Check sheet for the drawn part. Datum: minimum x, y, z corner. Units: mm. A direction names the side the tool comes from. Coordinates: 2 decimals unless noted, no trailing zeros. Order: outer loops, then holes, each group sorted by start corner. A loop starts at its lowest first (then second) coordinate and runs counter-clockwise, first axis right, second up.
Q1. Set-up check for the marked faces 4, 5 and 6: record each of +Z, -Z, +X, -X, +Y, -Y from which the full face is reachable in a straight line by a thin tool's end or side.
Q2. Depth check by flat-ended pin: P1, Ø12.5, axis at x = 62, z = 64, coming from the -Y side; P2, Ø7, axis at y = 41, z = 15, coming from the -X side; P3, Ø5.5, axis at x = 44, y = 22, coming from the +Z side (1 decimal). Enter the tip coordinate at first touch or a pass-through.
Q3. Cross-section at A-A, the plane x = 67. Record the boundary of the cut face in (y, z), and give its area (3 significant figures).
Q4. Thickness scan on line 1 (Y direction, x = 63, z = 83); line 2 (Z direction, x = 119, y = 13); line 3 (X direction, y = 12, z = 63) (1 decimal). Record the ranges inside material, lowest first.
Q5. Cross-section at B-B, the plane y = 46. Record the boundary of the cut face in (x, z), and give its area (3 significant figures).
Q6. Draft check along Z on the marked faces 1, 2 and 3. Enter one of: pulls with the +Z half, pulls with the -Z half, needs draft (parallel to the pull), parting line crosses it, or undercut.
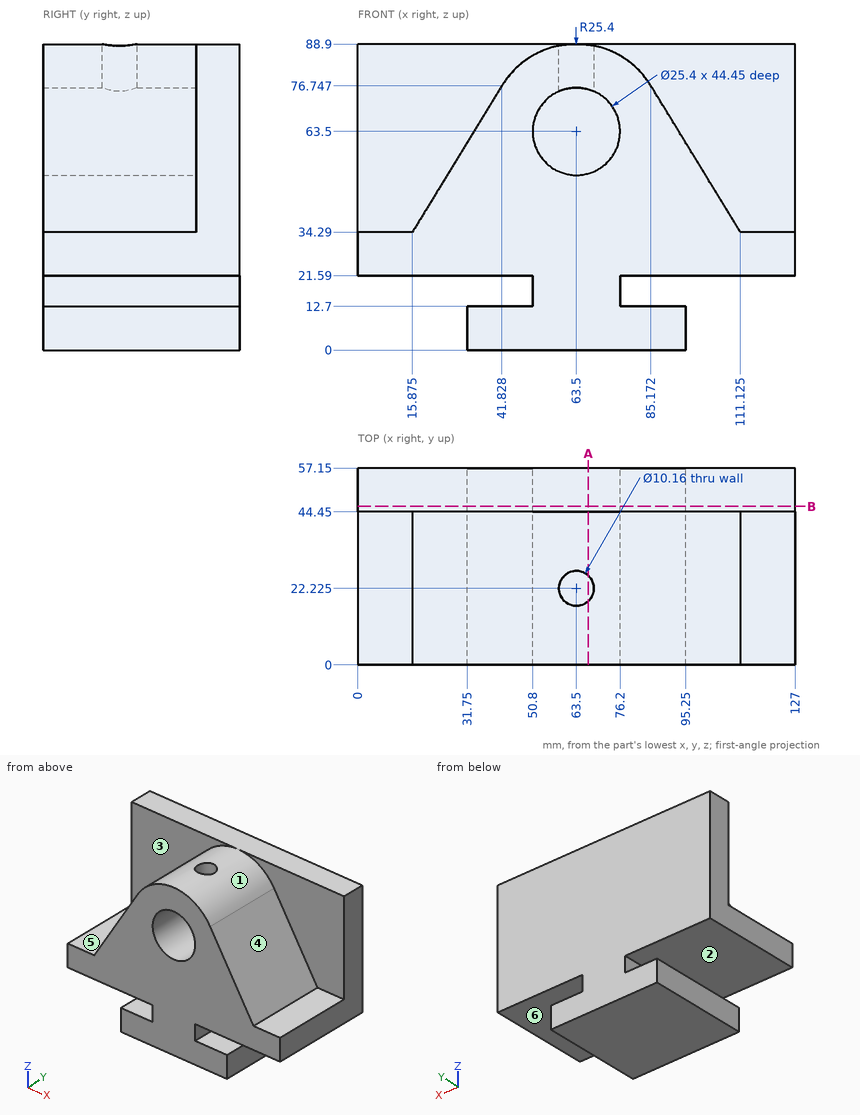
Check values:
1. face 4: +Z, +X, -Y
1. face 5: +Z, -X, -Y
1. face 6: +X, +Y, -Y
2. P1: stops at y = 44.45
2. P2: stops at x = 31.75
2. P3: stops at z = 82.6
3. outline: (0, 0) - (57.15, 0) - (57.15, 88.9) - (44.45, 88.9) - (44.45, 88.66) - (25.91, 88.66) - (25.91, 75.71) - (44.45, 75.71) - (44.45, 51.29) - (0, 51.29) - close; (0, 75.71) - (18.54, 75.71) - (18.54, 88.66) - (0, 88.66) - close
3. area: 3,890 mm2
4. line 1: y = 0 to 17.17, 27.28 to 57.15
4. line 2: z = 21.59 to 34.29
4. line 3: x = 33.4 to 50.8, 76.2 to 93.6
5. outline: (0, 21.59) - (50.8, 21.59) - (50.8, 12.7) - (31.75, 12.7) - (31.75, 0) - (95.25, 0) - (95.25, 12.7) - (76.2, 12.7) - (76.2, 21.59) - (127, 21.59) - (127, 88.9) - (0, 88.9) - close
5. area: 9,580 mm2
6. face 1: pulls with the +Z half
6. face 2: undercut
6. face 3: needs draft
